Read the model definition and answer for the solid it produces. Units are mm, in the model's axes. A direction names the side the tool comes from. Coordinates: 2 decimals unless noted, no trailing zeros. Order: outer loops, then holes, each group sorted by start corner. A loop starts at its lowest first (then second) coordinate and runs counter-clockwise, first axis right, second up. Notation, with made-up numbers: (-26.5, 61) -> (18.5, 61) arc R27 ccw to (18.5, 93) -> close; hole circle Ø6 at (-29.5, 58.25). An arc over 180 degrees is marked (long way). Return JSON: item names as keys, results as strings. Group by question number.
Autodesk Inventor part; units mm, degrees
ref_plane "YZ Plane" through (0, 0, 0) normal (1, 0, 0) x (0, 1, 0)
ref_plane "XZ Plane" through (0, 0, 0) normal (0, 1, 0) x (-1, 0, 0)
ref_plane "XY Plane" through (0, 0, 0) normal (0, 0, 1) x (1, 0, 0)
sketch "Boceto1" plane through (0, 0, 0) normal (0, 0, 1) x (1, 0, 0)
  line L0 (0, 0) -> (460, 0)
  line L1 (460, 0) -> (460, 40)
  line L2 (460, 40) -> (0, 40)
  line L3 (0, 40) -> (0, 0)
  dimension "d0" = 460
  dimension "d1" = 40
extrude "Placa1" add sketch "Boceto1" along normal blind 1
sketch "Boceto2" plane through (0, 39, 0) normal (0, 1, 0) x (-1, 0, 0)
  line L0 (-460, 0) -> (0, 0)
  line L1 (0, 0) -> (0, 50)
  line L2 (0, 50) -> (-460, 50)
  line L3 (-460, 50) -> (-460, 0)
edge flange "Pestaña1" height 50 angle 90 thickness 1 bend radius 1 thickness toward (0, 1, 0) relief tear relief width 1 relief depth 0.5 edges at (230, 40, 1) wall of the first edge with corners at (460, 39, 0) (0, 39, 0) (0, 39, 50) (460, 39, 50)
bend "Doblez1"
corner "Esquina1"
sketch "Boceto3" plane through (0, 0, 1) normal (0, 0, 1) x (1, 0, 0)
  circle A0 centre (23.3423, 20.935) radius 8.73
  circle A1 centre (436.5993, 20.935) radius 8.73
  line L0 (0, 0) -> (0, 38)
  line L1 (460, 40) -> (0, 40)
  dimension "d13" = 413.257
  dimension "d14" = 23.3423
  dimension "d15" = 17.46
  dimension "d16" = 17.46
  dimension "d17" = 19.065
extrude "Extrusión1" cut sketch "Boceto3" against normal blind 10
equation "\"d16\" = d15"
equation "\"d2\" = Grosor"
equation "\"d3\" = Anchura_desahogo_plegado"
equation "\"d4\" = Profundidad_desahogo_plegado"
equation "\"d5\" = Remanente_mínimo"
equation "\"d6\" = Radiodetransición"
equation "\"d9\" = Radio_pliegue"
equation "\"d10\" = Tamaño_destalonado"
equation "\"d11\" = TamañoSeparación"
equation "\"d12\" = Tamaño_de_radio_de_Jacobi"
equation "\"Radio_pliegue\" = Grosor"
equation "\"Anchura_desahogo_plegado\" = Grosor"
equation "\"Profundidad_desahogo_plegado\" = 0.5 * Grosor"
equation "\"Tamaño_destalonado\" = 4 * Grosor"
equation "\"Remanente_mínimo\" = 2 * Grosor"
equation "\"Radiodetransición\" = Radio_pliegue"
equation "\"Tamaño_de_radio_de_Jacobi\" = Radio_pliegue"
equation "\"TamañoSeparación\" = Grosor"
properties part number "perfil_fijacion"
1. Find section C-C on z = 32. Determine the outline of the cut face in (x, y).
2. Find section A-A on y = 17. Determine the outline of the cut face in (x, z).
3. Straight lines are drawn through the part: L1, parallel to Y at x = 181, z = 18.5; L2, parallel to Z at x = 76.5, y = 30. For each, find the intervals that lie inside material, in ascending order.
4. Given pin 1 (10 mm diameter, centred on x = 247, y = 33, fed in from +Z); pin 2 (14 mm diameter, centred on x = 23.34, y = 20.94, fed in from -Z), each flat-ended and moving along its own axis, determine where each tip first touches the part or whether it passes through.
5. For a pull along X with two mould halves and no side action, classify faces 1 (the face through (227, 19, 0)), 2 (the face through (16.414, 15.623, 0.507)), 3 (the face through (0, 39.4, 25.1)) as released by +X, released by -X, zero draft, split by the parting line, or undercut.
6. Find section B-B on x = 80. Determine the outline of the cut face in (y, z), and give its area (3 significant figures).
7. Find section D-D on y = 34. Determine the outline of the cut face in (x, z).
8. Which of the six approach directions +Z, -Z, +X, -X, +Y, -Y give full straight-line access (tool end or side, diameter ignored) to faces 4 (the face through (444.926, 23.557, 0.507)), 5 (the face through (227, 39, 26))?
Result:
{
 "1": {"outline": "(0, 39) -> (460, 39) -> (460, 40) -> (0, 40) -> close"},
 "2": {"outline": "(0, 0) -> (15.55, 0) -> (15.55, 1) -> (0, 1) -> close; (31.14, 0) -> (428.81, 0) -> (428.81, 1) -> (31.14, 1) -> close; (444.39, 0) -> (460, 0) -> (460, 1) -> (444.39, 1) -> close"},
 "3": {"L1": "39 to 40", "L2": "0 to 1"},
 "4": {"pin 1": "z = 1", "pin 2": "through"},
 "5": {"face 1": "zero draft", "face 2": "undercut", "face 3": "released by -X"},
 "6": {"outline": "(0, 0) -> (38, 0) arc R2 ccw to (40, 2) -> (40, 50) -> (39, 50) -> (39, 2) arc R1 cw to (38, 1) -> (0, 1) -> close", "area": "88.4 mm^2"},
 "7": {"outline": "(0, 0) -> (460, 0) -> (460, 1) -> (0, 1) -> close"},
 "8": {"face 4": "+Z, -Z", "face 5": "+Z, +X, -X, -Y"}
}
